Verification items for the finished model (mm, model axes). Give positions to 0.01 mm unless a question says otherwise; leave off trailing zeros. Loops run counter-clockwise (first coordinate to the right, second up) from the corner with the lowest first, then second, coordinate; pieces in that order, holes last. Notation, with made-up numbers: (7, 18) - (59, 18) arc R23 cw to (59, 32) - close; hole circle Ø2 at (25, -18). An arc over 180 degrees is marked (long way). Use one line per item in the form item = value.
```python
from build123d import *

# Parameters (mm, degrees)
BOSS_EXTRUDE1_DEPTH = 20
CUT_EXTRUDE1_REACH  = 444.747
SKETCH2_R           = 3


with BuildPart() as part:
    # Sketch1 → Boss-Extrude1 (new body)
    with BuildSketch(Plane(origin=(0, 0, 0), x_dir=(1, 0, 0), z_dir=(0, 1, 0))):
        Polygon((-225, -300), (225, -300), (225, -100), (325, -100), (325, 100), (225, 100), (225, 300), (-225, 300), (-225, 100), (-325, 100), (-325, -100), (-225, -100), align=None)
    extrude(amount=BOSS_EXTRUDE1_DEPTH)

    # Sketch2 → Cut-Extrude1 (cut, up to next)
    with BuildSketch(Plane(origin=(0, 20, 0), x_dir=(1, 0, 0), z_dir=(0, 1, 0)), mode=Mode.PRIVATE) as cut_extrude1_sk1:
        with Locations(Location((-295, -56, 0), (0, 0, 270))):
            Circle(SKETCH2_R)
    cut_extrude1_tool1 = extrude(cut_extrude1_sk1.sketch, amount=-CUT_EXTRUDE1_REACH, mode=Mode.PRIVATE) & part.part
    # Sketch2 → Cut-Extrude1 (cut, up to next)
    with BuildSketch(Plane(origin=(0, 20, 0), x_dir=(1, 0, 0), z_dir=(0, 1, 0)), mode=Mode.PRIVATE) as cut_extrude1_sk2:
        with Locations(Location((-263, -56, 0), (0, 0, 270))):
            Circle(SKETCH2_R)
    cut_extrude1_tool2 = extrude(cut_extrude1_sk2.sketch, amount=-CUT_EXTRUDE1_REACH, mode=Mode.PRIVATE) & part.part
    # Sketch2 → Cut-Extrude1 (cut, up to next)
    with BuildSketch(Plane(origin=(0, 20, 0), x_dir=(1, 0, 0), z_dir=(0, 1, 0)), mode=Mode.PRIVATE) as cut_extrude1_sk3:
        with Locations(Location((-263, 56, 0), (0, 0, 270))):
            Circle(SKETCH2_R)
    cut_extrude1_tool3 = extrude(cut_extrude1_sk3.sketch, amount=-CUT_EXTRUDE1_REACH, mode=Mode.PRIVATE) & part.part
    # Sketch2 → Cut-Extrude1 (cut, up to next)
    with BuildSketch(Plane(origin=(0, 20, 0), x_dir=(1, 0, 0), z_dir=(0, 1, 0)), mode=Mode.PRIVATE) as cut_extrude1_sk4:
        with Locations(Location((-295, 56, 0), (0, 0, 270))):
            Circle(SKETCH2_R)
    cut_extrude1_tool4 = extrude(cut_extrude1_sk4.sketch, amount=-CUT_EXTRUDE1_REACH, mode=Mode.PRIVATE) & part.part
    cut_extrude1_1 = cut_extrude1_tool1.solids().sort_by_distance((-295, 20, 56))[0]
    add(cut_extrude1_1, mode=Mode.SUBTRACT)
    cut_extrude1_2 = cut_extrude1_tool2.solids().sort_by_distance((-263, 20, 56))[0]
    add(cut_extrude1_2, mode=Mode.SUBTRACT)
    cut_extrude1_3 = cut_extrude1_tool3.solids().sort_by_distance((-263, 20, -56))[0]
    add(cut_extrude1_3, mode=Mode.SUBTRACT)
    cut_extrude1_4 = cut_extrude1_tool4.solids().sort_by_distance((-295, 20, -56))[0]
    add(cut_extrude1_4, mode=Mode.SUBTRACT)
    cut_extrude1 = cut_extrude1_1 + cut_extrude1_2 + cut_extrude1_3 + cut_extrude1_4  # Cut-Extrude1 as one shape, for the pattern or mirror that repeats it

    # Mirror1: Cut-Extrude1 across plane
    add(cut_extrude1.mirror(Plane(origin=(0, 0, 0), x_dir=(0, 0, 1), z_dir=(1, 0, 0))), mode=Mode.SUBTRACT)


solid = part.part
```
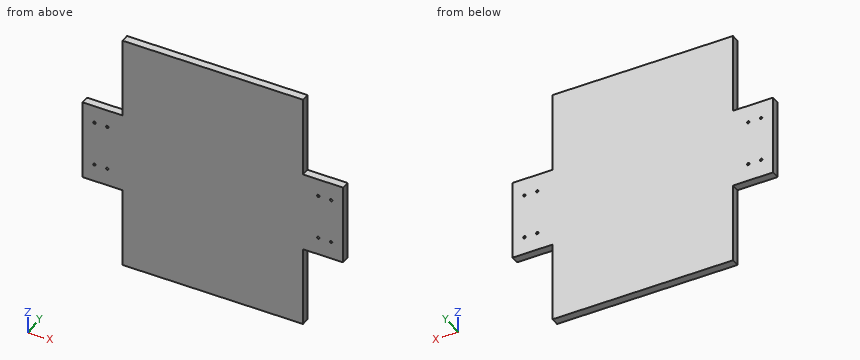
1. Depth check by flat-ended pin: pin 1 Ø3.5 at (x, z) = (-295, 56) entering from -Y; pin 2 Ø10 at (x, y) = (-288, 9) entering from -Z; pin 3 Ø1.5 at (y, z) = (15.5, -226) entering from +X; pin 4 Ø6 at (y, z) = (13, -225) entering from -X. Enter the tip coordinate at first touch or a pass-through.
Result set:
pin_1 = through
pin_2 = -100
pin_3 = 225
pin_4 = -225
2. Section check B-B, the plane z = 212. Record the cut outline in (x, y), then the cut area to 3 significant figures.
Result set:
outline = (-225, 0) - (225, 0) - (225, 20) - (-225, 20) - close
area = 9,000 mm²
3. Scan lines: probe 1 along X at (y, z) = (5, 56); probe 2 along Z at (x, y) = (263, 15.25); probe 3 along Z at (x, y) = (270.5, 18.5). Record each from-to range of solid material in increasing order.
Result set:
probe_1 = -325 to -298, -292 to -266, -260 to 260, 266 to 292, 298 to 325
probe_2 = -100 to -59, -53 to 53, 59 to 100
probe_3 = -100 to 100
4. Section check A-A, the plane y = 16.25. State how many separate pieces and enclosed holes the cut face has, then the cut area to 3 significant figures.
Result set:
separate_pieces = 1
enclosed_holes = 8
area = 310,000 mm²
